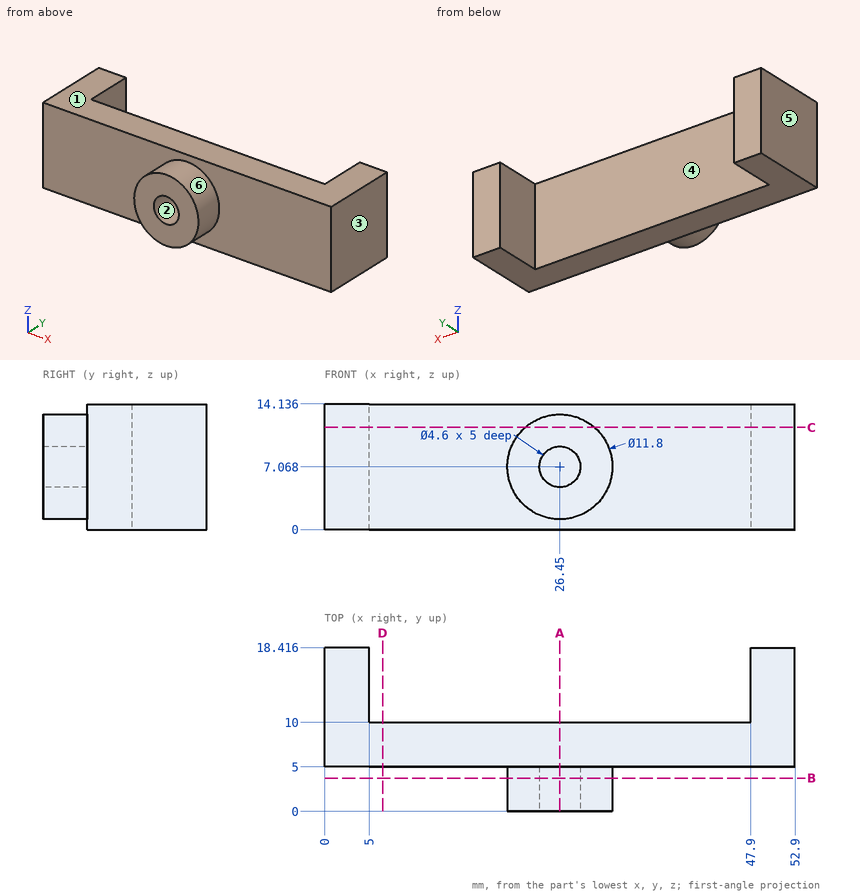
Part print with two shaded views. Sizes in mm from the minimum x, y, z corner. A direction names the side the tool comes from. Round coordinates to 2 decimals unless told otherwise and drop trailing zeros. Order: outer loops, then holes, each group sorted by start corner. A loop starts at its lowest first (then second) coordinate and runs counter-clockwise, first axis right, second up. Notation, with made-up numbers: (83, 3) - (121, 3) arc R19 ccw to (121, 23) - close; hole circle Ø11 at (81, 45.5). An arc over 180 degrees is marked (long way). Answer in a Markdown table with one row per item. Add a question column.
(1) Mould opens along X. For the marked faces 1, 2 and 3 say: +X half, -X half, draft (parallel to the pull), parting line (faces both ways), or undercut.
(2) Band-saw the part on D-D on x = 6.5. List the corners of the cut face in (y, z).
(3) Probe L1, parallel to X at y = 13.75, z = 10.25; L2, parallel to Y at x = 6, z = 12.5; L3, parallel to Y at x = 22.5, z = 5.75. List the from-to ranges inside material, lowest first. Write a range as [from, to].
(4) Drop flat-ended pins along their axis: pin 1 Ø7 at (x, z) = (14, 5.5) entering from -Y; pin 2 Ø1 at (x, z) = (17, 8.5) entering from +Y. Give the stop position or say it passes through.
(5) Band-saw the part on A-A on x = 26.45. List the corners of the cut face in (y, z).
(6) 3-axis set-ups, long thin cutter, end or side, ignore diameter. For the marked faces 4, 5 and 6: which of +Z, -Z, +X, -X, +Y, -Y reach the whole face in a straight line?
(7) Band-saw the part on B-B on y = 3.75. List the corners of the cut face in (x, z).
(8) Band-saw the part on C-C on z = 11.5. List the corners of the cut face in (x, y).
Data:
| question | item | result |
|---|---|---|
| 1 | face 1 | draft |
| 1 | face 2 | undercut |
| 1 | face 3 | +X half |
| 2 | outline | (5, 0) - (10, 0) - (10, 14.14) - (5, 14.14) - close |
| 3 | L1 | x = [0, 5], [47.9, 52.9] |
| 3 | L2 | y = [5, 10] |
| 3 | L3 | y = [0, 10] |
| 4 | pin 1 | stops at y = 5 |
| 4 | pin 2 | stops at y = 10 |
| 5 | outline | (0, 1.17) - (5, 1.17) - (5, 0) - (10, 0) - (10, 14.14) - (5, 14.14) - (5, 12.97) - (0, 12.97) - (0, 9.37) - (5, 9.37) - (5, 4.77) - (0, 4.77) - close |
| 6 | face 4 | +Z, -Z, +Y |
| 6 | face 5 | +Z, -Z, -X, +Y, -Y |
| 6 | face 6 | -Y |
| 7 | outline | circle Ø11.8 at (26.45, 7.07); hole circle Ø4.6 at (26.45, 7.07) |
| 8 | outline | (0, 5) - (22.56, 5) - (22.56, 0) - (30.34, 0) - (30.34, 5) - (52.9, 5) - (52.9, 18.42) - (47.9, 18.42) - (47.9, 10) - (5, 10) - (5, 18.42) - (0, 18.42) - close |
